from build123d import *
from build123d.topology import SkipClean

# Parameters (mm, degrees)
EXTRUDE_1_DEPTH     = 4
SKETCH_2_R          = 13.25
EXTRUDE_2_DEPTH     = 4
SKETCH_3_R          = 6
EXTRUDE_3_DEPTH     = 3.5
CUT_EXTRUDE_1_REACH = 31.327
SKETCH_4_R          = 4
FILLET_1_R          = 3
HOLE_WIZARD_1_D     = 5


with BuildPart() as part:
    # 草图1 → 凸台-拉伸1 (new body)
    with BuildSketch(Plane(origin=(0, 0, 0), x_dir=(1, 0, 0), z_dir=(0, 1, 0))):
        with BuildLine():
            Line((-3, 5), (-12.270391192, 5))
            ThreePointArc((-12.270391192, 5), (-13.25, 0), (-12.270391192, -5))
            Line((-12.270391192, -5), (-3, -5))
            Line((-3, -5), (-3, 5))
        make_face()
        with BuildLine():
            Line((-12.270391192, 5), (-23.5, 5))
            Line((-23.5, 5), (-23.5, -5))
            Line((-23.5, -5), (-12.270391192, -5))
            ThreePointArc((-12.270391192, -5), (-13.25, 0), (-12.270391192, 5))
        make_face()
        with BuildLine():
            ThreePointArc((12.270391192, 5), (0, 13.25), (-12.270391192, 5))
            Line((-12.270391192, 5), (-3, 5))
            Line((-3, 5), (-3, -5))
            Line((-3, -5), (-12.270391192, -5))
            ThreePointArc((-12.270391192, -5), (0, -13.25), (12.270391192, -5))
            Line((12.270391192, -5), (3, -5))
            Line((3, -5), (3, 5))
            Line((3, 5), (12.270391192, 5))
        make_face()
        with BuildLine():
            ThreePointArc((13.25, 0), (13.002791687, 2.547529853), (12.270391192, 5))
            Line((12.270391192, 5), (3, 5))
            Line((3, 5), (3, -5))
            Line((3, -5), (12.270391192, -5))
            ThreePointArc((12.270391192, -5), (13.002791687, -2.547529853), (13.25, 0))
        make_face()
        with BuildLine():
            Line((23.5, 5), (12.270391192, 5))
            ThreePointArc((12.270391192, 5), (13.002791687, 2.547529853), (13.25, 0))
            ThreePointArc((13.25, 0), (13.002791687, -2.547529853), (12.270391192, -5))
            Line((12.270391192, -5), (23.5, -5))
            Line((23.5, -5), (23.5, 5))
        make_face()
    extrude(amount=EXTRUDE_1_DEPTH)

    # 草图2 → 凸台-拉伸2 (add)
    with BuildSketch(Plane(origin=(0, 4, 0), x_dir=(1, 0, 0), z_dir=(0, 1, 0))):
        with Locations(Location((0, 0, 0), (0, 0, 22.170157164))):
            Circle(SKETCH_2_R)
    extrude(amount=EXTRUDE_2_DEPTH)

    # 草图3 → 凸台-拉伸3 (add)
    with SkipClean():  # the faces are left unmerged after this step: merging them gives an invalid solid
        with BuildSketch(Plane(origin=(0, 8, 0), x_dir=(1, 0, 0), z_dir=(0, 1, 0))):
            with Locations(Location((0, 0, 0), (0, 0, 270))):
                Circle(SKETCH_3_R)
        extrude(amount=EXTRUDE_3_DEPTH)

    # 草图4 → 切除-拉伸1 (cut, up to next)
    with BuildSketch(Plane(origin=(0, 11.5, 0), x_dir=(1, 0, 0), z_dir=(0, 1, 0)), mode=Mode.PRIVATE) as cut_extrude_1_sk1:
        with Locations(Location((0, 0, 0), (0, 0, 270))):
            Circle(SKETCH_4_R)
    cut_extrude_1_tool1 = extrude(cut_extrude_1_sk1.sketch, amount=-CUT_EXTRUDE_1_REACH, mode=Mode.PRIVATE) & part.part
    add(cut_extrude_1_tool1.solids().sort_by_distance((0, 11.5, 0))[0], mode=Mode.SUBTRACT)

    # 圆角1
    # the kernel refuses this fillet: 3 mm, written as the material it adds along each edge
    with BuildSketch(Plane(origin=(-12.270391192, 0, 5), x_dir=(-1, 0, 0), z_dir=(0, 1, 0))) as fillet_1_piece_1:
        with BuildLine():
            CenterArc((1.873953968, 3), FILLET_1_R, 209.492372675, 60.507627325)
            ThreePointArc((-0.737309754, 1.523076923), (-0.344316056, 0.773320696), (0, 0))
            Line((0, 0), (1.873953968, 0))
        make_face()
    extrude(amount=4)
    with BuildSketch(Plane(origin=(-12.270391192, 0, -5), x_dir=(0.43572231670003575, 0, -0.9000811423030447), z_dir=(0, 1, 0)), Plane(origin=(12.270391192, 0, 5), x_dir=(-0.4357223167001389, 0, 0.9000811423029949), z_dir=(0, 1, 0))) as fillet_1_piece_2:
        with BuildLine():
            CenterArc((1.883719863, 2.993877578), FILLET_1_R, 205.831264919, 60.507627325)
            Line((-0.816523564, 1.686710628), (0, 0))
            ThreePointArc((0, 0), (0.846077565, 0.027040696), (1.692155131, 0))
        make_face()
    extrude(amount=4)
    with BuildSketch(Plane(origin=(12.270391192, 0, -5), x_dir=(-0.43572231670013994, 0, -0.9000811423029943), z_dir=(0, 1, 0))) as fillet_1_piece_3:
        with BuildLine():
            CenterArc((1.883719863, -2.993877578), FILLET_1_R, 93.661107756, 60.507627325)
            Line((-0.816523564, -1.686710628), (0, 0))
            ThreePointArc((0, 0), (0.846077565, -0.027040696), (1.692155131, 0))
        make_face()
    extrude(amount=4)
    # the kernel refuses this fillet: 3 mm, written as the material it takes off along each edge
    with BuildSketch(Plane(origin=(-23.5, -7.5, 5), x_dir=(1, 0, 0), z_dir=(0, 1, 0)), Plane(origin=(23.5, -7.5, -5), x_dir=(-1, 0, 0), z_dir=(0, 1, 0)), Plane(origin=(23.5, -7.5, 5), x_dir=(0, 0, -1), z_dir=(0, 1, 0))) as fillet_1_2_piece_1:
        with BuildLine():
            CenterArc((FILLET_1_R, FILLET_1_R), FILLET_1_R, 180, 90)
            Line((0, FILLET_1_R), (0, 0))
            Line((0, 0), (FILLET_1_R, 0))
        make_face()
    extrude(amount=19, mode=Mode.SUBTRACT)
    with BuildSketch(Plane(origin=(-23.5, -7.5, -5), x_dir=(1, 0, 0), z_dir=(0, 1, 0))) as fillet_1_2_piece_2:
        with BuildLine():
            CenterArc((FILLET_1_R, -FILLET_1_R), FILLET_1_R, 90, 90)
            Line((0, -FILLET_1_R), (0, 0))
            Line((0, 0), (FILLET_1_R, 0))
        make_face()
    extrude(amount=19, mode=Mode.SUBTRACT)

    # 孔1 (through all)
    with Locations(Plane(origin=(0, 4, 0), x_dir=(1, 0, 0), z_dir=(0, 1, 0))):
        with Locations((-18.5, 0), (18.5, 0)):
            Hole(HOLE_WIZARD_1_D / 2)


solid = part.part
The model under review builds one solid part; all positions refer to its coordinate system, in mm. A direction names the side the tool comes from. Round coordinates to 2 decimals unless told otherwise and drop trailing zeros. Loops run counter-clockwise (first coordinate to the right, second up) from the corner with the lowest first, then second, coordinate; pieces in that order, holes last. Notation, with made-up numbers: (70, 30) -> (110, 30) arc R22 cw to (110, 55) -> close; hole circle Ø9 at (-2, 49.5). An arc over 180 degrees is marked (long way). Write item = value, one per line. Start each with the question number.
Item 1: For faces 4 (the flat face through (17, 2, -5)), 5 (the cylindrical face through (1.802, 9.726, 5.723)), 6 (the flat face through (-17, 2, 5)), list the 3-axis set-ups (+Z, -Z, +X, -X, +Y, -Y) from which the entire face can be reached by the end or side of a thin tool; tool diameter is ignored.
Item 2: Take a section at A-A on x = -20. Give the boundary of the cut face in (y, z), plus the area to 3 significant figures.
Item 3: Take a section at C-C on z = -3. Give the boundary of the cut face in (x, y), plus the area to 3 significant figures.
Item 4: Take a section at B-B on y = 2. Give the boundary of the cut face in (x, z).
Item 5: Insertion check: pin 1 (3 mm diameter, centred on x = -18.5, z = 0, fed in from +Y); pin 2 (6 mm diameter, centred on x = -10.5, y = 6, fed in from -Z); pin 3 (2 mm diameter, centred on x = -17.5, y = 3, fed in from -Z); pin 4 (13 mm diameter, centred on x = 17.5, z = 2.5, fed in from +Y). Each pin has a flat end and moves straight along its axis. Give the tip position at first contact, or say it passes through.
Item 6: Mouldability with a two-part tool opening along Z and no side actions: class faces 1 (the cylindrical face through (21, 2, 0)), 2 (the flat face through (17, 2, 5)), 3 (the cylindrical face through (12.61, 1.97, -5.42)) as released by +Z, released by -Z, zero draft, split by the parting line, or undercut.
Item 7: Take a section at D-D on x = -5. Give the boundary of the cut face in (y, z), plus the area to 3 significant figures.
Item 8: To check wall thickness, follow L1, parallel to Z at x = -18.5, y = 1; L2, parallel to X at y = 6.75, z = 0; L3, parallel to Z at x = 14.5, y = 2. State the ranges of each line that lie inside material, in increasing order.
Result:
q1.face_4 = -Z, +X, +Y, -Y
q1.face_5 = +Y
q1.face_6 = +Z, -X, +Y, -Y
q2.outline = (0, -5) -> (4, -5) -> (4, -2) -> (0, -2) -> close; (0, 2) -> (4, 2) -> (4, 5) -> (0, 5) -> close
q2.area = 24.0 mm²
q3.outline = (-23.33, 0) -> (-2.65, 0) -> (-2.65, 11.5) -> (-5.2, 11.5) -> (-5.2, 8) -> (-12.91, 8) -> (-12.91, 4) -> (-23.33, 4) -> close; (2.65, 0) -> (23.33, 0) -> (23.33, 4) -> (12.91, 4) -> (12.91, 8) -> (5.2, 8) -> (5.2, 11.5) -> (2.65, 11.5) -> close
q3.area = 265 mm²
q4.outline = (-23.5, -2) arc R3 ccw to (-20.5, -5) -> (-14.14, -5) arc R3 cw to (-11.53, -6.52) arc R13.25 ccw to (11.53, -6.52) arc R3 cw to (14.14, -5) -> (20.5, -5) arc R3 ccw to (23.5, -2) -> (23.5, 2) arc R3 ccw to (20.5, 5) -> (14.14, 5) arc R3 cw to (11.53, 6.52) arc R13.25 ccw to (-11.53, 6.52) arc R3 cw to (-14.14, 5) -> (-20.5, 5) arc R3 ccw to (-23.5, 2) -> close; hole circle Ø5 at (-18.5, 0); hole circle Ø8 at (0, 0); hole circle Ø5 at (18.5, 0)
q5.pin_1 = through
q5.pin_2 = -10.92
q5.pin_3 = -5
q5.pin_4 = 8
q6.face_1 = undercut
q6.face_2 = released by +Z
q6.face_3 = released by -Z
q7.outline = (0, -12.27) -> (8, -12.27) -> (8, -3.32) -> (11.5, -3.32) -> (11.5, 3.32) -> (8, 3.32) -> (8, 12.27) -> (0, 12.27) -> close
q7.area = 220 mm²
q8.L1 = -5 to -2.5, 2.5 to 5
q8.L2 = -13.25 to -4, 4 to 13.25
q8.L3 = -5 to 5
